Source: CAD feature listing. Evaluate the final solid. Frame: model axes, mm. Face numbers are marked on the shaded views. A direction names the side the tool comes from. Round coordinates to 2 decimals unless told otherwise and drop trailing zeros. Write each loop counter-clockwise with the first axis right and the second up, starting at its lowest first coordinate (ties: lowest second). Pieces come first, ordered by that corner, then holes.
from build123d import *

# Parameters (mm, degrees)
SKETCH_1_R          = 1.6
EXTRUDE_1_DEPTH     = 1
SKETCH_2_W          = 50
SKETCH_2_H          = 1
EXTRUDE_2_DEPTH     = 8.5
SKETCH_3_R          = 1.6
CUT_EXTRUDE_1_DEPTH = 10


with BuildPart() as part:
    # 草图1 → 凸台-拉伸1 (new body)
    with BuildSketch(Plane(origin=(0, 0, 0), x_dir=(1, 0, 0), z_dir=(0, 1, 0))):
        with BuildLine():
            Line((8, 0), (43, 0))
            Line((43, 0), (43, 9.7))
            Line((43, 9.7), (39, 9.7))
            ThreePointArc((39, 9.7), (33.5, 15.2), (39, 20.7))
            Line((39, 20.7), (50, 20.7))
            Line((50, 20.7), (50, 36))
            Line((50, 36), (0, 36))
            Line((0, 36), (0, 8))
            ThreePointArc((0, 8), (5.656854249, 5.656854249), (8, 0))
        make_face()
        with Locations(Location((8.5, 26, 0), (0, 0, 270))):
            Circle(SKETCH_1_R, mode=Mode.SUBTRACT)
        with Locations(Location((21.5, 4.4, 0), (0, 0, 270))):
            Circle(SKETCH_1_R, mode=Mode.SUBTRACT)
        with Locations(Location((34.5, 26, 0), (0, 0, 90))):
            Circle(SKETCH_1_R, mode=Mode.SUBTRACT)
        with Locations(Location((31.371170143, 6, 0), (0, 0, 270))):
            Circle(SKETCH_1_R, mode=Mode.SUBTRACT)
        with Locations(Location((11.628829857, 6, 0), (0, 0, 90))):
            Circle(SKETCH_1_R, mode=Mode.SUBTRACT)
    extrude(amount=EXTRUDE_1_DEPTH)

    # 草图2 → 凸台-拉伸2 (add)
    with BuildSketch(Plane(origin=(0, 1, 0), x_dir=(1, 0, 0), z_dir=(0, 1, 0))):
        with Locations((25, 35.5)):
            Rectangle(SKETCH_2_W, SKETCH_2_H)
    extrude(amount=EXTRUDE_2_DEPTH)

    # 草图3 → 切除-拉伸1 (cut)
    with BuildSketch(Plane.XY.offset(-35)):
        with Locations((46, 5)):
            Circle(SKETCH_3_R)
        with Locations((18, 5)):
            Circle(SKETCH_3_R)
    extrude(amount=-CUT_EXTRUDE_1_DEPTH, mode=Mode.SUBTRACT)


solid = part.part
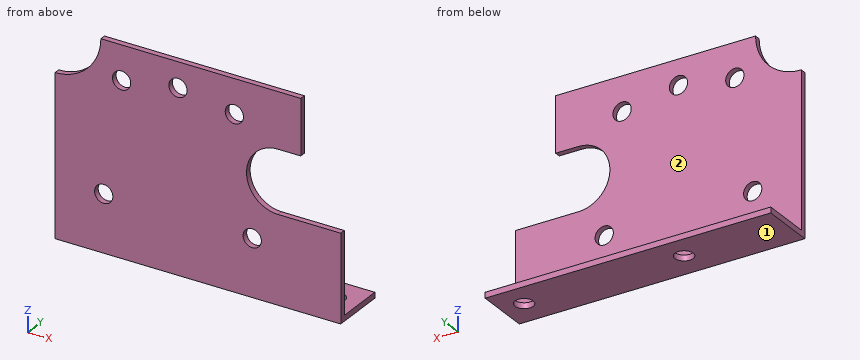
1) Section query D-D on x = 45.5. Return the cut outline in (y, z), then the cut area to 3 significant figures.
Taken from the geometry:
outline: (0, -36) - (3.48, -36) - (3.48, -35) - (1, -35) - (1, -20.7) - (0, -20.7) - close; (6.52, -36) - (9.5, -36) - (9.5, -35) - (6.52, -35) - close
area: 20.8 mm2
2) Section query C-C on z = -25.5. Return the cut outline in (x, y).
Taken from the geometry:
outline: (0, 0) - (6.98, 0) - (6.98, 1) - (0, 1) - close; (10.02, 0) - (32.98, 0) - (32.98, 1) - (10.02, 1) - close; (36.02, 0) - (50, 0) - (50, 1) - (36.02, 1) - close
3) Contact query for flat-ended pins moving along their axis: P1, Ø1, axis at x = 17, y = 3, coming from the +Z side; P2, Ø10, axis at x = 28, z = -15, coming from the +Y side; P3, Ø0.8, axis at x = 45, y = 0.5, coming from the +Z side. Output: stop coordinate, or through.
Taken from the geometry:
P1: stops at z = -35
P2: stops at y = 1
P3: stops at z = -20.7
4) Reachability of the marked faces 1 and 2 from +Z, -Z, +X, -X, +Y, -Y: full face, straight path, thin tool, end or side. Return the list, or none.
Taken from the geometry:
face 1: -Z, +X, -X, +Y, -Y
face 2: +Z, +X, -X, +Y
5) Material intervals for line 1 (X direction, y = 0.6, z = -26); line 2 (Z direction, x = 34.5, y = 0.4); line 3 (Z direction, x = 8.5, y = 4.75), sorted ascending.
Taken from the geometry:
line 1: x = 0 to 6.9, 10.1 to 32.9, 36.1 to 50
line 2: z = -36 to -27.6, -24.4 to -18.36, -12.04 to 0
line 3: z = -36 to -35
6) Section query A-A on x = 8.5. Return the cut outline in (y, z).
Taken from the geometry:
outline: (0, -36) - (9.5, -36) - (9.5, -35) - (1, -35) - (1, -27.6) - (0, -27.6) - close; (0, -24.4) - (1, -24.4) - (1, 0) - (0, 0) - close
7) Section query B-B on y = 5. Return the cut outline in (x, z).
Taken from the geometry:
outline: (0, -36) - (16.4, -36) - (16.4, -35) - (0, -35) - close; (19.6, -36) - (44.4, -36) - (44.4, -35) - (19.6, -35) - close; (47.6, -36) - (50, -36) - (50, -35) - (47.6, -35) - close
